```python
from build123d import *

# Parameters (mm, degrees)
ESQUISSE1_W             = 30
ESQUISSE1_H             = 19
BOSS_EXTRU_1_DEPTH      = 16
ESQUISSE2_R             = 3
ENL_V_MAT_EXTRU_2_DEPTH = 29
ESQUISSE3_R             = 1
ENL_V_MAT_EXTRU_3_DEPTH = 8
ESQUISSE7_W             = 28
ESQUISSE7_H             = 17
ENL_V_MAT_EXTRU_4_DEPTH = 15
ESQUISSE8_R             = 2
ENL_V_MAT_EXTRU_7_DEPTH = 1.5


with BuildPart() as part:
    # Esquisse1 → Boss.-Extru.1 (new body)
    with BuildSketch(Plane.XY):
        with Locations((15, 9.5)):
            Rectangle(ESQUISSE1_W, ESQUISSE1_H)
    extrude(amount=BOSS_EXTRU_1_DEPTH)

    # Esquisse2 → Enlèv. mat.-Extru.2 (cut)
    with BuildSketch(Plane.ZY):
        with Locations((8, 9.5)):
            Circle(ESQUISSE2_R)
    extrude(amount=-ENL_V_MAT_EXTRU_2_DEPTH, mode=Mode.SUBTRACT)

    # Esquisse3 → Enlèv. mat.-Extru.3 (cut)
    with BuildSketch(Plane(origin=(30, 0, 0), x_dir=(0, 0, -1), z_dir=(1, 0, 0))):
        with Locations((-8, 9.5)):
            Circle(ESQUISSE3_R)
    extrude(amount=-ENL_V_MAT_EXTRU_3_DEPTH, mode=Mode.SUBTRACT)

    # Esquisse7 → Enlèv. mat.-Extru.4 (cut)
    with BuildSketch(Plane(origin=(0, 0, 0), x_dir=(-1, 0, 0), z_dir=(0, 0, -1))):
        with Locations((-15, 9.5)):
            Rectangle(ESQUISSE7_W, ESQUISSE7_H)
    extrude(amount=-ENL_V_MAT_EXTRU_4_DEPTH, mode=Mode.SUBTRACT)

    # Esquisse8 → Enlèv. mat.-Extru.7 (cut)
    with BuildSketch(Plane(origin=(0, 19, 0), x_dir=(1, 0, 0), z_dir=(0, 1, 0))):
        with Locations(Location((23, -13, 0), (0, 0, 270))):
            Circle(ESQUISSE8_R)
        with Locations(Location((11, -3, 0), (0, 0, 270))):
            Circle(ESQUISSE8_R)
    extrude(amount=-ENL_V_MAT_EXTRU_7_DEPTH, mode=Mode.SUBTRACT)


solid = part.part
```
Here's how the part is built. I have some questions about the finished solid (model axes, mm). A direction names the side the tool comes from. Give positions to 0.01 mm unless a question says otherwise; leave off trailing zeros. Loops run counter-clockwise (first coordinate to the right, second up) from the corner with the lowest first, then second, coordinate; pieces in that order, holes last. Notation, with made-up numbers: M -38.5,26 L -27.5,26 A35 cw -27.5,62 Z; hole C -23,58.25 d8. An arc over 180 degrees is marked long. Put each result on its own line as item: value. Start each with the question number.
(1) I want a section at A-A on y = 9.5. Please give me the cut outline in (x, z), then the cut area to 3 significant figures.
(2) Will these pins go through, and if not, where does the flat tip stop? pin 1 Ø3.5 at (x, z) = (23, 13) entering from +Y; pin 2 Ø1.5 at (x, y) = (6, 8) entering from -Z; pin 3 Ø3.5 at (y, z) = (9.5, 8) entering from -X.
(3) I need wall thicknesses on line 1 along Y through (x, z) = (29.7, 8); line 2 along Y through (x, z) = (24, 5.25); line 3 along X through (y, z) = (13.5, 3.75). Which ranges of each line are inside material? Lowest first, please. Write a range as [from, to].
(4) I want a section at C-C on y = 15. Please give me the cut outline in (x, z).
(5) For faces 1 (the cylindrical face through (0.49, 8.35, 10.77)), 2 (the flat face through (13.8, 0.4, 0)), 3 (the flat face through (15, 18, 7)), 4 (the cylindrical face through (12.983, 18.507, 2.74)), which set-ups out of +Z, -Z, +X, -X, +Y, -Y let a thin tool reach every point of the face, with its end or its side?
(6) I want a section at D-D on x = 14.25. Please give me the cut outline in (y, z).
(7) If we mould it in two halves opening along Y, with no side actions, what happens to faces 5 (the cylindrical face through (21.8, 18.5, 11.4)), 6 (the flat face through (15, 0, 8)), 7 (the flat face through (15, 19, 8)), 8 (the flat face through (1, 7, 6))? For each: +Y half, -Y half, draft (parallel to the pull), parting line (faces both ways), or undercut.
(8) I want a section at B-B on z = 3. Please give me the cut outline in (x, y), then the cut area to 3 significant figures.
Answer block:
1. outline: M 0,0 L 1,0 L 1,5 L 0,5 Z; M 0,11 L 1,11 L 1,15 L 29,15 L 29,9 L 30,9 L 30,16 L 0,16 Z; M 29,0 L 30,0 L 30,7 L 29,7 Z
1. area: 52.0 mm^2
2. pin 1: y = 1
2. pin 2: z = 15
2. pin 3: x = 29
3. line 1: [0, 8.5], [10.5, 19]
3. line 2: [0, 1], [18, 19]
3. line 3: [0, 1], [29, 30]
4. outline: M 0,0 L 1,0 L 1,15 L 29,15 L 29,0 L 30,0 L 30,16 L 0,16 Z
5. face 1: -X
5. face 2: -Z, +X, -X, +Y, -Y
5. face 3: -Z
5. face 4: +Y
6. outline: M 0,0 L 1,0 L 1,15 L 18,15 L 18,0 L 19,0 L 19,16 L 0,16 Z
7. face 5: draft
7. face 6: -Y half
7. face 7: +Y half
7. face 8: undercut
8. outline: M 0,0 L 30,0 L 30,19 L 13,19 L 13,18 L 29,18 L 29,1 L 1,1 L 1,18 L 9,18 L 9,19 L 0,19 Z
8. area: 90.0 mm^2
